CAD build for the part. Positions are in the model's coordinates, mm. Face numbers are marked on the shaded views. A direction names the side the tool comes from. Give positions to 0.01 mm unless a question says otherwise; leave off trailing zeros. Order: outer loops, then holes, each group sorted by start corner. A loop starts at its lowest first (then second) coordinate and runs counter-clockwise, first axis right, second up. Notation, with made-up numbers: (9.5, 22.25) -> (40.5, 22.25) arc R13 cw to (40.5, 43.25) -> close; hole circle Ø9 at (-27, 79.25). An arc over 180 degrees is marked (long way). Answer as CSV lines item,"result".
```python
from build123d import *

# Parameters (mm, degrees)
SCHIZZO1_W                                           = 11
SCHIZZO1_H                                           = 9.5
SCHIZZO2_R                                           = 4.75
ESTRUSIONE_ESTRUSIONE1_DEPTH                         = 3.5
FORO_PER_VITE_M2_1_D                                 = 2.459
FORO_PER_VITE_M2_1_DEPTH                             = 13
FORO_LAMATO_PER_VITE_M3_5_A_TESTA_ESAGON_D           = 4
FORO_LAMATO_PER_VITE_M3_5_A_TESTA_ESAGON_DEPTH       = 13
FORO_LAMATO_PER_VITE_M3_5_A_TESTA_ESAGON_CBORE_D     = 8
FORO_LAMATO_PER_VITE_M3_5_A_TESTA_ESAGON_CBORE_DEPTH = 8.5
SCHIZZO7_W                                           = 1.2295
SCHIZZO7_H                                           = 11.749995321
SMUSSO1_SIZE                                         = 0.3


with BuildPart() as part:
    # Schizzo1 → Rivoluzione1 (revolve)
    with BuildSketch(Plane(origin=(0, 0, 0), x_dir=(-1, 0, 0), z_dir=(0, 0, -1))):
        with Locations((-5.5, 8.25)):
            Rectangle(SCHIZZO1_W, SCHIZZO1_H)
    revolve(axis=Axis((0, 3.5, 0), (0, 1, 0)))

    # Schizzo2 → Estrusione-Estrusione1 (add)
    with BuildSketch(Plane.XZ.offset(-3.5)):
        Circle(SCHIZZO2_R)
    extrude(amount=ESTRUSIONE_ESTRUSIONE1_DEPTH)

    # Foro per Vite M2-1
    with Locations(Plane(origin=(0, 13, 0), x_dir=(1, 0, 0), z_dir=(0, 1, 0))):
        with Locations((0, 8), (-8, 0), (0, -8), (8, 0)):
            Hole(FORO_PER_VITE_M2_1_D / 2, depth=FORO_PER_VITE_M2_1_DEPTH)

    # Foro lamato per Vite M3.5 a testa esagonale-1
    with Locations(Plane(origin=(0, 13, 0), x_dir=(1, 0, 0), z_dir=(0, 1, 0))):
        with Locations((0, 0)):
            CounterBoreHole(FORO_LAMATO_PER_VITE_M3_5_A_TESTA_ESAGON_D / 2, FORO_LAMATO_PER_VITE_M3_5_A_TESTA_ESAGON_CBORE_D / 2, FORO_LAMATO_PER_VITE_M3_5_A_TESTA_ESAGON_CBORE_DEPTH, depth=FORO_LAMATO_PER_VITE_M3_5_A_TESTA_ESAGON_DEPTH)

    # Schizzo7 → Foro per Vite M2-2 (revolve, cut)
    with BuildSketch(Plane(origin=(-2.69149863, 10, 2.69149863), x_dir=(-0.707106781, 0, -0.707106781), z_dir=(0, 1, 0))):
        with Locations((0.61475, 5.874997661)):
            Rectangle(SCHIZZO7_W, SCHIZZO7_H)
    revolve(axis=Axis((1.798629431, 10, -1.798629431), (-0.707106781, 0, 0.707106781)), mode=Mode.SUBTRACT)

    # Smusso1
    smusso1_edges = [part.edges().sort_by_distance(p)[0] for p in [
        (-11, 13, 0),
        (-11, 3.5, 0),
        (-4.75, 0, 0),
    ]]
    chamfer(smusso1_edges, length=SMUSSO1_SIZE)


solid = part.part
```
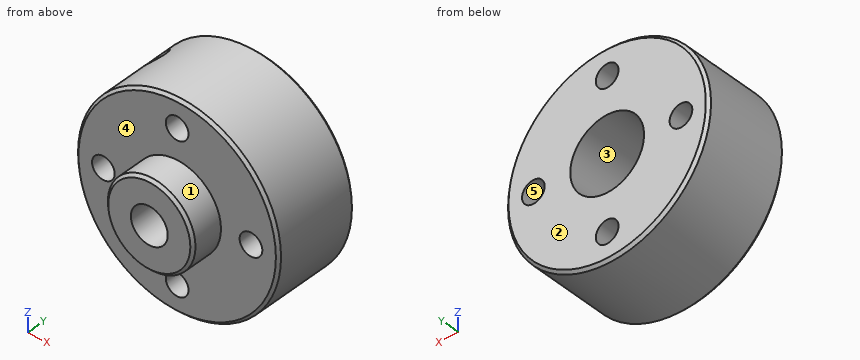
1) Wall check: line 1 along Z through (x, y) = (0, 10.25); line 2 along X through (y, z) = (11.5, -0.75); line 3 along X through (y, z) = (9.5, 1). Give the ranges that are in metal, low to high. Write a range as [from, to].
Data:
line 1,"z = [-11, -9.23], [-6.77, -4], [4, 6.77], [9.23, 11]"
line 2,"x = [-10.97, -8.97], [-7.03, -3.93], [3.93, 7.03], [8.97, 10.97]"
line 3,"x = [-10.95, -8.72], [-7.28, -3.87], [3.87, 7.28], [8.72, 10.95]"
2) Pull direction Z, two halves, no side cores. Call the marked faces 1, 2 and 3: pulls with the +Z half, pulls with the -Z half, needs draft (parallel to the pull), parting line crosses it, or undercut.
Data:
face 1,"parting line crosses it"
face 2,"needs draft"
face 3,"undercut"
3) Pin check, flat tips, straight feed: P1, Ø3.5, axis at x = 0, z = 0, coming from the +Y side; P2, Ø4, axis at x = -8, z = 0, coming from the -Y side; P3, Ø4, axis at y = 4.5, z = 4.5, coming from the +X side. Stop position of each tip, or through.
Data:
P1,"passes through"
P2,"stops at y = 3.5"
P3,"stops at x = 10.71"
4) Band-saw the part on A-A, the plane x = 0. Give the number of separate pieces and of enclosed holes in the cut face, then the cut area to 3 significant figures.
Data:
separate pieces,"4"
enclosed holes,"0"
area,"109 mm2"
5) Which spindle directions (+Z, -Z, +X, -X, +Y, -Y) get a long thin tool onto all of the face, cutting with end or side? Do the marked faces 4 and 5. Say none if no direction does.
Data:
face 4,"-Y"
face 5,"+Y, -Y"
6) Band-saw the part on C-C, the plane y = 11.5. Write the cut outline in (x, z).
Data:
outline,"circle Ø22 at (0, 0); hole circle Ø2.46 at (-8, 0); hole circle Ø8 at (0, 0); hole circle Ø2.46 at (0, -8); hole circle Ø2.46 at (0, 8); hole circle Ø2.46 at (8, 0)"
7) Band-saw the part on D-D, the plane y = 2.25. Write the cut outline in (x, z), then the cut area to 3 significant figures.
Data:
outline,"circle Ø9.5 at (0, 0); hole circle Ø4 at (0, 0)"
area,"58.3 mm2"
